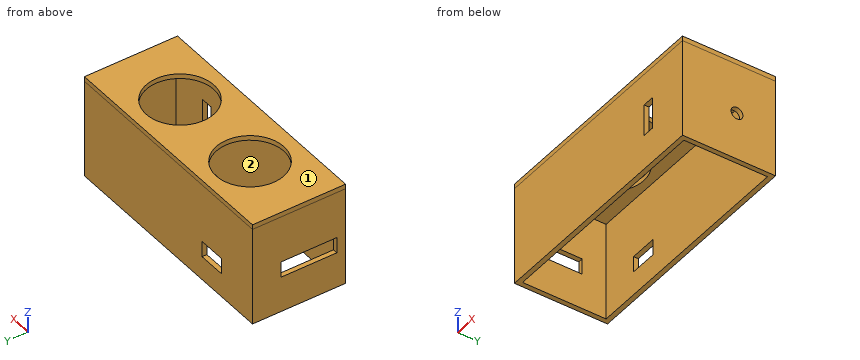
from build123d import *

# Parameters (mm, degrees)
F_3DSKETCH1_R       = 8.5
BOSS_EXTRUDE3_DEPTH = 1.2
SKETCH3_W           = 60
SKETCH3_H           = 23.4
SKETCH3_W_2         = 57.6
SKETCH3_H_2         = 21
BOSS_EXTRUDE4_DEPTH = 26
SKETCH6_W           = 3
SKETCH6_H           = 8
CUT_EXTRUDE1_DEPTH  = 4
SKETCH7_W           = 7
SKETCH7_H           = 4
CUT_EXTRUDE2_DEPTH  = 4
CUT_EXTRUDE4_DEPTH  = 4
SKETCH10_W          = 4
SKETCH10_H          = 4.5
SKETCH10_H_2        = 9.5
CUT_EXTRUDE5_DEPTH  = 4


with BuildPart() as part:
    # 3DSketch1 → Boss-Extrude3 (new body)
    with BuildSketch(Plane(origin=(-25.740687228, -9.071236551, 0), x_dir=(0.9316545551067793, 0.3633452764916439, 0), z_dir=(0, 0, -1))):
        Polygon((0, 0), (55.899273306, 21.800716589), (64.401552776, 0), (8.50227947, -21.800716589), align=None)
        with Locations(Location((20.555094449, -4.541815956, 0), (0, 0, 21.305783618))):
            Circle(F_3DSKETCH1_R, mode=Mode.SUBTRACT)
        with Locations(Location((43.846458327, 4.541815956, 0), (0, 0, 21.305783618))):
            Circle(F_3DSKETCH1_R, mode=Mode.SUBTRACT)
    extrude(amount=BOSS_EXTRUDE3_DEPTH)

    # Sketch3 → Boss-Extrude4 (add)
    with BuildSketch(Plane.XY):
        with Locations((4.259312772, 2.628763449)):
            Rectangle(SKETCH3_W, SKETCH3_H)
        with Locations((4.259312772, 2.628763449)):
            Rectangle(SKETCH3_W_2, SKETCH3_H_2, mode=Mode.SUBTRACT)
    extrude(amount=-BOSS_EXTRUDE4_DEPTH)

    # Sketch6 → Cut-Extrude1 (cut)
    with BuildSketch(Plane.XZ.offset(9.071236551)):
        with Locations((22.059312772, -13.2)):
            Rectangle(SKETCH6_W, SKETCH6_H)
    extrude(amount=-CUT_EXTRUDE1_DEPTH, mode=Mode.SUBTRACT)

    # Sketch7 → Cut-Extrude2 (cut)
    with BuildSketch(Plane(origin=(0, 14.328763449, 0), x_dir=(1, 0, 0), z_dir=(0, 1, 0))):
        with Locations((-11.240687228, 18)):
            Rectangle(SKETCH7_W, SKETCH7_H)
    extrude(amount=-CUT_EXTRUDE2_DEPTH, mode=Mode.SUBTRACT)

    # Sketch9 → Cut-Extrude4 (cut)
    with BuildSketch(Plane(origin=(34.259312772, 0, 0), x_dir=(0, 0, -1), z_dir=(1, 0, 0))):
        with BuildLine():
            Line((12.5, 4.628763449), (14, 4.628763449))
            Line((14, 4.628763449), (15.5, 4.628763449))
            ThreePointArc((15.5, 4.628763449), (14, 6.128763449), (12.5, 4.628763449))
        make_face()
        with BuildLine():
            Line((15.5, 4.628763449), (14, 4.628763449))
            Line((14, 4.628763449), (12.5, 4.628763449))
            ThreePointArc((12.5, 4.628763449), (14, 3.128763449), (15.5, 4.628763449))
        make_face()
    extrude(amount=-CUT_EXTRUDE4_DEPTH, mode=Mode.SUBTRACT)

    # Sketch10 → Cut-Extrude5 (cut)
    with BuildSketch(Plane.ZY.offset(25.740687228)):
        with Locations((-15, 4.878763449)):
            Rectangle(SKETCH10_W, SKETCH10_H)
        with Locations((-15, -2.121236551)):
            Rectangle(SKETCH10_W, SKETCH10_H_2)
    extrude(amount=-CUT_EXTRUDE5_DEPTH, mode=Mode.SUBTRACT)


solid = part.part
The listing builds one solid part. Answer for the finished solid, in the listing's coordinates (mm). Face numbers are marked on the shaded views. Coordinates: 2 decimals unless noted, no trailing zeros. Write each loop counter-clockwise with the first axis right and the second up, starting at its lowest first coordinate (ties: lowest second). Pieces come first, ordered by that corner, then holes. Notation, with made-up numbers: (69.5, 16.5) -> (87.5, 16.5) arc R22 cw to (87.5, 54.5) -> close; hole circle Ø4 at (48, 20.5). An arc over 180 degrees is marked (long way). One line per question, with ' | ' between items.
1. Given pin 1 Ø10.5 at (x, y) = (5, 1) entering from -Z, flat-ended and moving along its own axis, determine where the tip first touches the part or whether it passes through.
Verdict:
pin 1: stops at z = -1.2
2. Section A-A (z = -14) is taken. Determine the outline of the cut face in (x, y), and give its area (3 significant figures).
Verdict:
outline: (-25.74, -9.07) -> (20.56, -9.07) -> (20.56, -7.87) -> (-24.54, -7.87) -> (-24.54, -6.87) -> (-25.74, -6.87) -> close; (-25.74, 7.13) -> (-24.54, 7.13) -> (-24.54, 13.13) -> (33.06, 13.13) -> (33.06, 6.13) -> (34.26, 6.13) -> (34.26, 14.33) -> (-25.74, 14.33) -> close; (23.56, -9.07) -> (34.26, -9.07) -> (34.26, 3.13) -> (33.06, 3.13) -> (33.06, -7.87) -> (23.56, -7.87) -> close | area: 170 mm^2
3. For a pull along X with two mould halves and no side action, classify the marked faces 1 and 2 as released by +X, released by -X, zero draft, split by the parting line, or undercut.
Verdict:
face 1: zero draft | face 2: undercut
4. Section B-B (x = -9) is taken. Determine the outline of the cut face in (y, z), and give its area (3 significant figures).
Verdict:
outline: (-9.07, -26) -> (-7.87, -26) -> (-7.87, -1.2) -> (-5.84, -1.2) -> (-5.84, 0) -> (-9.07, 0) -> close; (11.09, -1.2) -> (13.13, -1.2) -> (13.13, -16) -> (14.33, -16) -> (14.33, 0) -> (11.09, 0) -> close; (13.13, -26) -> (14.33, -26) -> (14.33, -20) -> (13.13, -20) -> close | area: 62.5 mm^2
5. Straight lines are drawn through the part: line 1 (Y direction, x = 7, z = -4.25); line 2 (X direction, y = 5.5, z = -19.25); line 3 (Y direction, x = 33.8, z = -14). For each, find the intervals that lie inside material, in ascending order.
Verdict:
line 1: y = -9.07 to -7.87, 13.13 to 14.33 | line 2: x = -25.74 to -24.54, 33.06 to 34.26 | line 3: y = -9.07 to 3.13, 6.13 to 14.33
6. Section D-D (z = -2.75) is taken. Determine the outline of the cut face in (x, y).
Verdict:
outline: (-25.74, -9.07) -> (34.26, -9.07) -> (34.26, 14.33) -> (-25.74, 14.33) -> close; hole (-24.54, -7.87) -> (33.06, -7.87) -> (33.06, 13.13) -> (-24.54, 13.13) -> close
7. Section C-C (y = -5.25) is taken. Determine the outline of the cut face in (x, z), and give its area (3 significant figures).
Verdict:
outline: (-25.74, -26) -> (-24.54, -26) -> (-24.54, -17) -> (-25.74, -17) -> close; (-25.74, -13) -> (-24.54, -13) -> (-24.54, -1.2) -> (-11.43, -1.2) -> (-11.43, 0) -> (-25.74, 0) -> close; (-5.05, -1.2) -> (13.57, -1.2) -> (13.57, 0) -> (-5.05, 0) -> close; (19.95, -1.2) -> (33.06, -1.2) -> (33.06, -26) -> (34.26, -26) -> (34.26, 0) -> (19.95, 0) -> close | area: 111 mm^2
